from build123d import *

# Parameters (mm, degrees)
F1_DEPTH = 12
F2_R     = 1.99999


# Not quite as in the source:
# - a fillet or chamfer is up to 0.001 mm smaller than in the source, because OpenCascade refuses the exact size
# - a feature names something its author has since deleted; it is built from what else it names


with BuildPart() as f1:
    # F0 (on Top) → F1 (new body)
    with BuildSketch(Plane.XY):
        with BuildLine():
            Line((2, 14.3612188522), (0, 14.3612188522))
            Line((0, 14.3612188522), (0, 11.6508584444))
            ThreePointArc((0, 11.6508584444), (0.4713307349, 10.3612188522), (0, 9.0715792599))
            Line((0, 9.0715792599), (0, 6.3612188522))
            Line((0, 6.3612188522), (2, 6.3612188522))
            Line((2, 6.3612188522), (2, 14.3612188522))
        make_face()
        with BuildLine():
            Line((0, 11.6508584444), (0, 14.3612188522))
            Line((0, 14.3612188522), (-1.5286692651, 14.3612188522))
            ThreePointArc((-1.5286692651, 14.3612188522), (-5.4053887158, 11.346635668), (-3.4387615336, 6.8467420026))
            ThreePointArc((-3.4387615336, 6.8467420026), (-2.9444425376, 6.8562954182), (-2.7, 7.2860516088))
            Line((-2.7, 7.2860516088), (-2.7, 8.7401129613))
            ThreePointArc((-2.7, 8.7401129613), (-2.9949681852, 11.7213539472), (0, 11.6508584444))
        make_face()
    extrude(amount=F1_DEPTH)

    # F2 (radius 2 in the source; OpenCascade refuses exactly that, so slightly less here)
    f2_edges = [f1.edges().sort_by_distance(p)[0] for p in [
        (0, 6.361219, 6),
    ]]
    fillet(f2_edges, radius=F2_R)


solid = f1.part
The model under review builds one solid part; all positions refer to its coordinate system, in mm. Round coordinates to 2 decimals unless told otherwise and drop trailing zeros. Loops run counter-clockwise (first coordinate to the right, second up) from the corner with the lowest first, then second, coordinate; pieces in that order, holes last. Notation, with made-up numbers: (87.5, 32.25) - (105.5, 32.25) arc R16 ccw to (105.5, 60.25) - close; hole circle Ø1 at (-28, 74). An arc over 180 degrees is marked (long way). Use CSV: the item, a comma, the result in double quotes.
(1) Take a section at D-D, the plane y = 13.5. Give the boundary of the cut face in (x, z), plus the area to 3 significant figures.
Working result:
outline,"(-4.01, 0) - (2, 0) - (2, 12) - (-4.01, 12) - close"
area,"72.1 mm^2"
(2) Clearance check with flat-ended pins moving along their axes: P1, Ø1, axis at y = 11.5, z = 4, coming from the -X side; P2, Ø3, axis at x = -4.5, z = 9.5, coming from the +Y side. State where each tip first meets the part, or that it passes through.
Working result:
P1,"stops at x = -5.48"
P2,"stops at y = 14.08"
(3) For line 1 (Y direction, x = -1.5, z = 4); line 2 (X direction, y = 7.75, z = 7); line 3 (X direction, y = 9.5, z = 10.5), list the stretches that pass through material, from the lowest coordinate up.
Working result:
line 1,"y = 12.36 to 14.36"
line 2,"x = -4.56 to -2.7, 0.1 to 2"
line 3,"x = -5.43 to -3.33, 0.28 to 2"
(4) Take a section at A-A, the plane y = 10. Give the boundary of the cut face in (x, z), plus the area to 3 significant figures.
Working result:
outline,"(-5.51, 0) - (-3.5, 0) - (-3.5, 12) - (-5.51, 12) - close; (0.44, 0) - (2, 0) - (2, 12) - (0.44, 12) - close"
area,"42.9 mm^2"
(5) The part is to be moulded in two halves that separate along X. For faces 1 (the flat face through (2, 10, 6)), 2 (the flat face through (-2.7, 8, 6)), 3 (the cylindrical face through (0.57, 6.963, 6.084)), 4 (the flat face through (0, 14.361, 6)), say which applies: pulls with the +X half, pulls with the -X half, needs draft (parallel to the pull), parting line crosses it, or undercut.
Working result:
face 1,"pulls with the +X half"
face 2,"undercut"
face 3,"undercut"
face 4,"needs draft"
(6) Take a section at C-C, the plane x = 0.25. Give the boundary of the cut face in (y, z), plus the area to 3 significant figures.
Working result:
outline,"(7.39, 0) - (9.45, 0) - (9.45, 12) - (7.39, 12) - close; (11.28, 0) - (14.36, 0) - (14.36, 12) - (11.28, 12) - close"
area,"61.7 mm^2"
